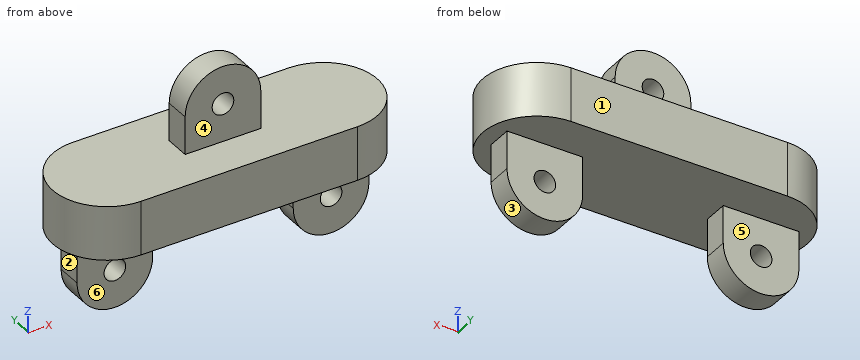
from build123d import *

# Parameters (mm, degrees)
BOSS_EXTRUDE1_DEPTH = 5
SKETCH3_W           = 7
SKETCH3_H           = 2.333333334
BOSS_EXTRUDE2_DEPTH = 3.5
SKETCH6_W           = 3.5
SKETCH6_H           = 2.333333334
REVOLVE1_ANGLE      = 180
CUT_EXTRUDE1_REACH  = 8.167
SKETCH7_R           = 1
SKETCH8_W           = 7
SKETCH8_H           = 2.33
BOSS_EXTRUDE3_DEPTH = 3.5
SKETCH9_W           = 3.5
SKETCH9_H           = 2.33
REVOLVE2_ANGLE      = 180
SKETCH9_3_W         = 3.5
SKETCH9_3_H         = 2.33
REVOLVE3_ANGLE      = 180
CUT_EXTRUDE2_REACH  = 8.165
SKETCH11_R          = 1


with BuildPart() as part:
    # Sketch2 → Boss-Extrude1 (new body)
    with BuildSketch(Plane.XY):
        with BuildLine():
            Line((-10, -5), (10, -5))
            ThreePointArc((10, -5), (15, 0), (10, 5))
            Line((10, 5), (-10, 5))
            ThreePointArc((-10, 5), (-15, 0), (-10, -5))
        make_face()
    extrude(amount=-BOSS_EXTRUDE1_DEPTH)

    # Sketch3 → Boss-Extrude2 (add)
    with BuildSketch(Plane.XY):
        Rectangle(SKETCH3_W, SKETCH3_H)
    extrude(amount=BOSS_EXTRUDE2_DEPTH)

    # Sketch6 → Revolve1 (revolve)
    with BuildSketch(Plane.XY.offset(3.5)):
        with Locations((-1.75, 0)):
            Rectangle(SKETCH6_W, SKETCH6_H)
    revolve(axis=Axis((0, 1.166666667, 3.5), (0, 1, 0)), revolution_arc=REVOLVE1_ANGLE)

    # Sketch7 → Cut-Extrude1 (cut, up to next)
    with BuildSketch(Plane(origin=(0, 1.166666667, 0), x_dir=(1, 0, 0), z_dir=(0, 1, 0)), mode=Mode.PRIVATE) as cut_extrude1_sk1:
        with Locations((0, -3.5)):
            Circle(SKETCH7_R)
    cut_extrude1_tool1 = extrude(cut_extrude1_sk1.sketch, amount=-CUT_EXTRUDE1_REACH, mode=Mode.PRIVATE) & part.part
    add(cut_extrude1_tool1.solids().sort_by_distance((0, 1.166667, 3.5))[0], mode=Mode.SUBTRACT)

    # Sketch8 → Boss-Extrude3 (add)
    with BuildSketch(Plane(origin=(0, 0, -5), x_dir=(-1, 0, 0), z_dir=(0, 0, -1))):
        with Locations((-10, 0)):
            Rectangle(SKETCH8_W, SKETCH8_H)
        with Locations((10, 0)):
            Rectangle(SKETCH8_W, SKETCH8_H)
    extrude(amount=BOSS_EXTRUDE3_DEPTH)

    # Sketch9 → Revolve2 (revolve)
    with BuildSketch(Plane(origin=(0, 0, -8.5), x_dir=(-1, 0, 0), z_dir=(0, 0, -1))):
        with Locations((-11.75, 0)):
            Rectangle(SKETCH9_W, SKETCH9_H)
    revolve(axis=Axis((10, 1.165, -8.5), (0, 1, 0)), revolution_arc=REVOLVE2_ANGLE)

    # Sketch9_3 → Revolve3 (revolve)
    with BuildSketch(Plane(origin=(0, 0, -8.5), x_dir=(-1, 0, 0), z_dir=(0, 0, -1))):
        with Locations((8.25, 0)):
            Rectangle(SKETCH9_3_W, SKETCH9_3_H)
    revolve(axis=Axis((-10, 1.165, -8.5), (0, 1, 0)), revolution_arc=REVOLVE3_ANGLE)

    # Sketch11 → Cut-Extrude2 (cut, up to next)
    with BuildSketch(Plane(origin=(0, 1.165, 0), x_dir=(1, 0, 0), z_dir=(0, 1, 0)), mode=Mode.PRIVATE) as cut_extrude2_sk1:
        with Locations((-10, 8.5)):
            Circle(SKETCH11_R)
    cut_extrude2_tool1 = extrude(cut_extrude2_sk1.sketch, amount=-CUT_EXTRUDE2_REACH, mode=Mode.PRIVATE) & part.part
    add(cut_extrude2_tool1.solids().sort_by_distance((-10, 1.165, -8.5))[0], mode=Mode.SUBTRACT)
    # Sketch11 → Cut-Extrude2 (cut, up to next)
    with BuildSketch(Plane(origin=(0, 1.165, 0), x_dir=(1, 0, 0), z_dir=(0, 1, 0)), mode=Mode.PRIVATE) as cut_extrude2_sk2:
        with Locations((10, 8.5)):
            Circle(SKETCH11_R)
    cut_extrude2_tool2 = extrude(cut_extrude2_sk2.sketch, amount=-CUT_EXTRUDE2_REACH, mode=Mode.PRIVATE) & part.part
    add(cut_extrude2_tool2.solids().sort_by_distance((10, 1.165, -8.5))[0], mode=Mode.SUBTRACT)


solid = part.part
CAD build for the part. Positions are in the model's coordinates, mm. Face numbers are marked on the shaded views. A direction names the side the tool comes from. Round coordinates to 2 decimals unless told otherwise and drop trailing zeros. Order: outer loops, then holes, each group sorted by start corner. A loop starts at its lowest first (then second) coordinate and runs counter-clockwise, first axis right, second up. Notation, with made-up numbers: (52, -23.75) - (81, -23.75) arc R12 ccw to (81, -3.75) - close; hole circle Ø1 at (-4, 70.25). An arc over 180 degrees is marked (long way). Return JSON: item names as keys, results as strings.
(1) Wall check: probe 1 along X at (y, z) = (0.4, -8.5); probe 2 along Z at (x, y) = (-10, -0.4); probe 3 along Z at (x, y) = (0, -0.4). Give the ranges that are in metal, low to high. Write a range as from..to.
Answer key:
{"probe 1": "x = -13.5..-11, -9..-6.5, 6.5..9, 11..13.5", "probe 2": "z = -12..-9.5, -7.5..0", "probe 3": "z = -5..2.5, 4.5..7"}
(2) Cut at A-A (x = 0). Give the cut face in (y, z), then the cut area to 3 significant figures.
Answer key:
{"outline": "(-5, -5) - (5, -5) - (5, 0) - (1.17, 0) - (1.17, 2.5) - (-1.17, 2.5) - (-1.17, 0) - (-5, 0) - close; (-1.17, 4.5) - (1.17, 4.5) - (1.17, 7) - (-1.17, 7) - close", "area": "61.7 mm^2"}
(3) Cut at B-B (y = 0). Give the cut face in (x, z), then the cut area to 3 significant figures.
Answer key:
{"outline": "(-15, -5) - (-13.5, -5) - (-13.5, -8.5) arc R3.5 ccw to (-6.5, -8.5) - (-6.5, -5) - (6.5, -5) - (6.5, -8.5) arc R3.5 ccw to (13.5, -8.5) - (13.5, -5) - (15, -5) - (15, 0) - (3.5, 0) - (3.5, 3.5) arc R3.5 ccw to (-3.5, 3.5) - (-3.5, 0) - (-15, 0) - close; hole circle Ø2 at (-10, -8.5); hole circle Ø2 at (0, 3.5); hole circle Ø2 at (10, -8.5)", "area": "272 mm^2"}
(4) Cut at C-C (z = -3.75). Give the cut face in (x, y).
Answer key:
{"outline": "(-10, -5) - (10, -5) arc R5 ccw to (10, 5) - (-10, 5) arc R5 ccw to start"}
(5) Cut at D-D (x = -12.25). Give the cut face in (y, z) (3 decimals).
Answer key:
{"outline": "(-4.465, -5) - (-1.165, -5) - (-1.165, -11.181) - (1.165, -11.181) - (1.165, -5) - (4.465, -5) - (4.465, 0) - (-4.465, 0) - close"}
(6) Pull direction X, two halves, no side cores. Call the marked faces 1, 2 and 3: +X half, -X half, draft (parallel to the pull), parting line (faces both ways), or undercut.
Answer key:
{"face 1": "draft", "face 2": "-X half", "face 3": "undercut"}
(7) Tool access for the marked faces 4, 5 and 6: list every direction of +Z, -Z, +X, -X, +Y, -Y with a clear straight run to the whole face (end or side of a thin tool).
Answer key:
{"face 4": "+Z, +X, -X, -Y", "face 5": "-Z, +X, -X, +Y", "face 6": "-Z, +X, -X, -Y"}
(8) Pin check, flat tips, straight feed: pin 1 Ø1.2 at (y, z) = (0, -7.5) entering from -X; pin 2 Ø0.7 at (y, z) = (0, -7.5) entering from +X; pin 3 Ø0.7 at (y, z) = (-0.5, 1.5) entering from -X; pin 4 Ø1.8 at (x, z) = (10, -8.5) entering from -Y. Stop position of each tip, or through.
Answer key:
{"pin 1": "stops at x = -13.5", "pin 2": "stops at x = 13.5", "pin 3": "stops at x = -3.5", "pin 4": "passes through"}
